```python
from build123d import *

# Parameters (mm, degrees)
BOSS_EXTRUDE1_DEPTH     = 8.382
FILLET1_R               = 25.4
FILLET2_R               = 3.175
FILLET3_R               = 6.35
SHELL1_T                = 2.54
CUT_EXTRUDE1_DEPTH      = 46.914035814
CUT_EXTRUDE1_DEPTH_BACK = 46.914035814
SKETCH2_W               = 9.652
SKETCH2_H               = 10.16
SKETCH3_R               = 1.397
BOSS_EXTRUDE2_DEPTH     = 16.764
SKETCH4_R               = 2.921
BOSS_EXTRUDE3_DEPTH     = 1.27
FILLET4_R               = 3.175
CUT_EXTRUDE2_DEPTH      = 47.162775769
CUT_EXTRUDE2_DEPTH_BACK = 47.162775769
SKETCH5_W               = 7.62
SKETCH5_H               = 15.24
SKETCH6_R               = 5.08
BOSS_EXTRUDE4_DEPTH     = 16.764
SKETCH7_R               = 4.318
BOSS_EXTRUDE5_DEPTH     = 1.27
CHAMFER1_SIZE           = 1.27
SKETCH9_W               = 16.764
SKETCH9_H               = 12.7
CUT_EXTRUDE3_DEPTH      = 3.81
FILLET5_R               = 0.762


# Some blends are built 0.0001 mm under size
with BuildPart() as part:
    # Sketch1 → Boss-Extrude1 (new, symmetric)
    with BuildSketch(Plane.XY):
        with BuildLine():
            Line((3.931691361, -1.785196639), (12.7, 17.526))
            Line((12.7, 17.526), (15.24, 38.354))
            Line((15.24, 38.354), (0, 44.704))
            Line((0, 44.704), (-15.24, 38.354))
            Line((-15.24, 38.354), (-12.7, 17.526))
            Line((-12.7, 17.526), (-3.931691361, -1.785196639))
            ThreePointArc((-3.931691361, -1.785196639), (0, -4.318), (3.931691361, -1.785196639))
        make_face()
    extrude(amount=BOSS_EXTRUDE1_DEPTH, both=True)

    # Fillet1
    fillet1_edges = [part.edges().sort_by_distance(p)[0] for p in [
        (0, 44.704, 0),
    ]]
    fillet(fillet1_edges, radius=FILLET1_R)

    # Fillet2
    fillet2_edges = [part.edges().sort_by_distance(p)[0] for p in [
        (-15.24, 38.354, 0),
        (15.24, 38.354, 0),
    ]]
    fillet(fillet2_edges, radius=FILLET2_R)

    # Fillet3
    fillet3_edges = [part.edges().sort_by_distance(p)[0] for p in [
        (-12.7, 17.526, 0),
        (12.7, 17.526, 0),
    ]]
    fillet(fillet3_edges, radius=FILLET3_R)

    # Shell1 (no face opened: a closed hollow body)
    add(offset(amount=-SHELL1_T, mode=Mode.PRIVATE), mode=Mode.SUBTRACT)

    # Sketch2 → Cut-Extrude1 (cut, two sides: drawn at the far end of the back side and taken through both)
    with BuildSketch(Plane(origin=(0, 0, 0), x_dir=(0, 0, -1), z_dir=(1, 0, 0)).offset(-CUT_EXTRUDE1_DEPTH_BACK)):
        with Locations((0, 0.762)):
            Rectangle(SKETCH2_W, SKETCH2_H)
    extrude(amount=CUT_EXTRUDE1_DEPTH + CUT_EXTRUDE1_DEPTH_BACK, mode=Mode.SUBTRACT)

    # Sketch3 → Boss-Extrude2 (add)
    with BuildSketch(Plane.XY.offset(8.382)):
        Circle(SKETCH3_R)
    extrude(amount=-BOSS_EXTRUDE2_DEPTH)

    # Sketch4 → Boss-Extrude3 (add)
    with BuildSketch(Plane.XY.offset(8.382)):
        Circle(SKETCH4_R)
    boss_extrude3 = extrude(amount=BOSS_EXTRUDE3_DEPTH)

    # Mirror1: Boss-Extrude3 across plane
    add(boss_extrude3.mirror(Plane.XY))

    # Fillet4
    # the kernel refuses this fillet: 3.175 mm, written as the material it takes off along each edge
    with BuildSketch(Plane(origin=(0, 0, 9.652), x_dir=(1, 0, 0), z_dir=(0, -1, 0))) as fillet4_piece_1:
        with BuildLine():
            CenterArc((0.381, -3.175), FILLET4_R, 36.869897646, 53.130102354)
            Line((0.381, 0), (0.381, 0.0635))
            Line((0.381, 0.0635), (2.921, 0.0635))
            Line((2.921, 0.0635), (2.9845, 0))
            ThreePointArc((2.9845, 0), (2.9845, -0.635), (2.9718, -1.2319))
            Line((2.9718, -1.2319), (2.921, -1.27))
        make_face()
    revolve(axis=Axis((0, 0, 9.652), (0, 0, 1)), mode=Mode.SUBTRACT)
    with BuildSketch(Plane(origin=(0, 0, -9.652), x_dir=(1, 0, 0), z_dir=(0, -1, 0))) as fillet4_piece_2:
        with BuildLine():
            CenterArc((0.381, 3.175), FILLET4_R, 270, 53.130102354)
            Line((0.381, 0), (0.381, -0.0635))
            Line((0.381, -0.0635), (2.921, -0.0635))
            Line((2.921, -0.0635), (2.9845, 0))
            ThreePointArc((2.9845, 0), (2.9845, 0.635), (2.9718, 1.2319))
            Line((2.9718, 1.2319), (2.921, 1.27))
        make_face()
    revolve(axis=Axis((0, 0, -9.652), (0, 0, 1)), mode=Mode.SUBTRACT)

    # Sketch5 → Cut-Extrude2 (cut, two sides: drawn at the far end of the back side and taken through both)
    with BuildSketch(Plane(origin=(0, 0, 0), x_dir=(0, 0, -1), z_dir=(1, 0, 0)).offset(-CUT_EXTRUDE2_DEPTH_BACK)):
        with Locations((0, 27.347333333)):
            Rectangle(SKETCH5_W, SKETCH5_H)
    extrude(amount=CUT_EXTRUDE2_DEPTH + CUT_EXTRUDE2_DEPTH_BACK, mode=Mode.SUBTRACT)

    # Sketch6 → Boss-Extrude4 (add)
    with BuildSketch(Plane.XY.offset(8.382)):
        with Locations((0, 28.575)):
            Circle(SKETCH6_R)
    extrude(amount=-BOSS_EXTRUDE4_DEPTH)

    # Sketch7 → Boss-Extrude5 (add)
    with BuildSketch(Plane.XY.offset(8.382)):
        with Locations((0, 28.575)):
            Circle(SKETCH7_R)
    boss_extrude5 = extrude(amount=BOSS_EXTRUDE5_DEPTH)

    # Mirror2: Boss-Extrude5 across plane
    add(boss_extrude5.mirror(Plane.XY))

    # Chamfer1
    chamfer1_edges = [part.edges().sort_by_distance(p)[0] for p in [
        (-4.318, 28.575, 9.652),
        (-4.318, 28.575, -9.652),
    ]]
    chamfer(chamfer1_edges, length=CHAMFER1_SIZE - 0.0001)  # a hair under: the kernel refuses the full size

    # Sketch9 → Cut-Extrude3 (cut, symmetric)
    with BuildSketch(Plane.XY):
        with Locations((0, 44.809833333)):
            Rectangle(SKETCH9_W, SKETCH9_H)
    extrude(amount=CUT_EXTRUDE3_DEPTH, both=True, mode=Mode.SUBTRACT)

    # Fillet5
    fillet5_edges = [part.edges().sort_by_distance(p)[0] for p in [
        (-11.393675882, 39.956635049, -8.382),
        (-11.393675882, 39.956635049, 8.382),
        (0, 42.587333333, -8.382),
        (0, 42.587333333, 8.382),
        (11.393675882, 39.956635049, -8.382),
        (11.393675882, 39.956635049, 8.382),
        (-13.88335447, 27.229506655, -8.382),
        (-14.540660788, 37.946752783, -8.382),
        (14.540660788, 37.946752783, -8.382),
        (-13.88335447, 27.229506655, 8.382),
        (-14.540660788, 37.946752783, 8.382),
        (14.540660788, 37.946752783, 8.382),
        (0, -4.318, 8.382),
        (13.88335447, 27.229506655, -8.382),
        (13.88335447, 27.229506655, 8.382),
        (-8.114190115, 7.426278367, -8.382),
        (-12.628279179, 17.546141938, -8.382),
        (12.628279179, 17.546141938, -8.382),
        (-8.114190115, 7.426278367, 8.382),
        (-12.628279179, 17.546141938, 8.382),
        (12.628279179, 17.546141938, 8.382),
        (8.114190115, 7.426278367, 8.382),
        (8.114190115, 7.426278367, -8.382),
        (0, -4.318, -8.382),
    ]]
    fillet(fillet5_edges, radius=FILLET5_R)


solid = part.part
```
The listing builds one solid part. Answer for the finished solid, in the listing's coordinates (mm). A direction names the side the tool comes from. Round coordinates to 2 decimals unless told otherwise and drop trailing zeros. Use CSV: the item, a comma, the result in double quotes. Start each with the question number.
(1) Section A-A on z = -1.75 is taken. Count the separate pieces of the cut face and the enclosed holes in it, then the cut area to 3 significant figures.
(2) The mould has two halves that part along Y. Classify faces 1 (the face through (-6.79, 10.65, 0.08)), 2 (the face through (-6, 5.842, 0)), 3 (the face through (2, -2, -4.826)): released by +Y, released by -Y, zero draft, split by the parting line, or undercut.
(3) Which of the six approach directions +Z, -Z, +X, -X, +Y, -Y give full straight-line access (tool end or side, diameter ignored) to faces 4 (the face through (6.67, 10.39, 0.08)), 5 (the face through (3, 24, 8.382)), 6 (the face through (3, 24, -8.382))?
(4) Each of these flat-tipped pins is pushed along its axis until it touches: pin 1 (1 mm diameter, centred on y = 21.5, z = -5.5, fed in from +X); pin 2 (0.8 mm diameter, centred on x = 11.5, z = -1, fed in from +Y); pin 3 (3 mm diameter, centred on x = -13.5, z = 0.5, fed in from -Y); pin 4 (8 mm diameter, centred on x = 0, y = 2, fed in from -Z). Where does it stop, or does it pass through?
(5) Consider L1, parallel to Z at x = 9.75, y = 33; L2, parallel to X at y = 27, z = -5.75; L3, parallel to Z at x = -3.25, y = 0.5. Determine where each line is inside the solid, lowest interval first. Write a range as from..to.
A:
1,separate pieces,"6"
1,enclosed holes,"0"
1,area,"205 mm²"
2,face 1,"undercut"
2,face 2,"released by -Y"
2,face 3,"zero draft"
3,face 4,"none"
3,face 5,"+Z"
3,face 6,"-Z"
4,pin 1,"stops at x = 13.25"
4,pin 2,"stops at y = 40.08"
4,pin 3,"stops at y = 15.98"
4,pin 4,"stops at z = -9.65"
5,L1,"z = -8.38..-5.84, 5.84..8.38"
5,L2,"x = -13.86..-11.3, -4.83..4.83, 11.3..13.86"
5,L3,"z = -8.38..-4.83, 4.83..8.38"
